from build123d import *

# Parameters (mm, degrees)
F1_DEPTH = 50.8
F2_R     = 12.7
F4_D     = 12.7


with BuildPart() as f1:
    # F0 (on Top) → F1 (new body)
    with BuildSketch(Plane.XY):
        Polygon((0, 50.8), (0, 0), (152.4, 0), (152.4, 76.2), (101.6, 76.2), (101.6, 50.8), align=None)
    extrude(amount=F1_DEPTH)

    # F2
    f2_edges = [f1.edges().sort_by_distance(p)[0] for p in [
        (152.4, 76.2, 25.4),
        (152.4, 0, 25.4),
        (50.8, 50.8, 0),
        (0, 50.8, 25.4),
        (0, 0, 25.4),
    ]]
    fillet(f2_edges, radius=F2_R)

    # F4 (through all)
    with Locations(Plane.XY.offset(50.8)):
        with Locations((50.8, 25.4), (101.6, 25.4)):
            Hole(F4_D / 2)


solid = f1.part
CAD build for the part. Positions are in the model's coordinates, mm. A direction names the side the tool comes from. Give positions to 0.01 mm unless a question says otherwise; leave off trailing zeros. Loops run counter-clockwise (first coordinate to the right, second up) from the corner with the lowest first, then second, coordinate; pieces in that order, holes last. Notation, with made-up numbers: M 7.5,57.5 L 42.5,57.5 A19 cw 42.5,83.5 Z; hole C 70,48.25 d5. An arc over 180 degrees is marked long. One line per question, with ' | ' between items. Start each with the question number.
1. Saw through at A-A on z = 40. Give the cut face in (x, y), plus the area to 3 significant figures.
2. Saw through at B-B on y = 25.4. Give the cut face in (x, z).
3. 3-axis set-ups, long thin cutter, end or side, ignore diameter. For faces 5 (the face through (50.09, 47.18, 3.82)), 6 (the face through (58, 50.8, 31)), 7 (the face through (3.62, 3.82, 25.76)): which of +Z, -Z, +X, -X, +Y, -Y reach the whole face in a straight line?
4. Flat gauge pins, fed straight in: pin 1 (11.5 mm diameter, centred on x = 44.5, z = 34, fed in from +Y); pin 2 (19 mm diameter, centred on y = 52.5, z = 24.5, fed in from -X). Where does each tip first touch, or does it go through?
5. Saw through at C-C on x = 50.8. Give the cut face in (y, z), plus the area to 3 significant figures.
6. Two-plate mould, pull along Y, no slides. Class faces 1 (the face through (148.78, 72.38, 25.76)), 2 (the face through (148.58, 3.62, 25.76)), 3 (the face through (44.934, 22.968, 25.044)), 4 (the face through (0, 26, 25)): pulls with the +Y half, pulls with the -Y half, needs draft (parallel to the pull), parting line crosses it, or undercut.
7. Probe L1, parallel to X at y = 26, z = 23; L2, parallel to Y at x = 50.8, z = 28; L3, parallel to X at y = 51.5, z = 18. List the from-to ranges inside material, lowest first. Write a range as from..to.
8. Saw through at D-D on x = 72.5. Give the cut face in (y, z).
Result sheet:
1) outline: M 0,12.7 A12.7 ccw 12.7,0 L 139.7,0 A12.7 ccw 152.4,12.7 L 152.4,63.5 A12.7 ccw 139.7,76.2 L 101.6,76.2 L 101.6,50.8 L 12.7,50.8 A12.7 ccw 0,38.1 Z; hole C 50.8,25.4 d12.7; hole C 101.6,25.4 d12.7 | area: 8,640 mm^2
2) outline: M 0,0 L 44.45,0 L 44.45,50.8 L 0,50.8 Z; M 57.15,0 L 95.25,0 L 95.25,50.8 L 57.15,50.8 Z; M 107.95,0 L 152.4,0 L 152.4,50.8 L 107.95,50.8 Z
3) face 5: -Z, -X, +Y | face 6: +Z, -Z, -X, +Y | face 7: +Z, -Z, -X, -Y
4) pin 1: stops at y = 50.8 | pin 2: stops at x = 0.98
5) outline: M 0,0 L 19.05,0 L 19.05,50.8 L 0,50.8 Z; M 31.75,0 L 38.1,0 A12.7 ccw 50.8,12.7 L 50.8,50.8 L 31.75,50.8 Z | area: 1,900 mm^2
6) face 1: pulls with the +Y half | face 2: pulls with the -Y half | face 3: undercut | face 4: needs draft
7) L1: x = 0..44.48, 57.12..95.28, 107.92..152.4 | L2: y = 0..19.05, 31.75..50.8 | L3: x = 101.6..152.4
8) outline: M 0,0 L 38.1,0 A12.7 ccw 50.8,12.7 L 50.8,50.8 L 0,50.8 Z
